Autodesk Inventor part; units mm, degrees
ref_plane "YZ Plane" through (0, 0, 0) normal (1, 0, 0) x (0, 1, 0)
ref_plane "XZ Plane" through (0, 0, 0) normal (0, 1, 0) x (-1, 0, 0)
ref_plane "XY Plane" through (0, 0, 0) normal (0, 0, 1) x (1, 0, 0)
sketch "Sketch1" plane through (0, 0, 0) normal (0, 1, 0) x (-1, 0, 0)
  line L0 (0, 0) -> (-165, 0)
  line L1 (-165, 0) -> (-165, 100)
  line L2 (0, 0) -> (0, 100)
  line L3 (0, 100) -> (-165, 100)
  dimension "d0" = 165
  dimension "d1" = 100
extrude "Extrusion1" add sketch "Sketch1" along normal blind 3
chamfer "Chamfer1" distance 2 angle 45 4 edges at (165, 1.5, 100) (165, 1.5, 0) (0, 1.5, 100) (0, 1.5, 0)
sketch "Sketch2" plane through (0, 0, 0) normal (0, -1, 0) x (1, 0, 0)
  line L0 (163, 100) -> (165, 98)
  line L1 (165, 98) -> (135, 98)
  line L2 (135, 98) -> (135, 74.7)
  line L3 (135, 98) -> (90, 98)
  line L4 (135, 74.7) -> (90, 74.7)
  line L5 (90, 74.7) -> (90, 98)
  line L6 (89, 73.7) -> (136, 73.7)
  line L7 (136, 73.7) -> (136, 99)
  line L8 (136, 99) -> (89, 99)
  line L9 (89, 99) -> (89, 73.7)
  line L10 (165, 98) -> (165, 2)
  line L11 (165, 2) -> (135, 2)
  line L12 (135, 2) -> (135, 25.3)
  line L13 (135, 25.3) -> (90, 25.3)
  line L14 (90, 25.3) -> (90, 2)
  line L15 (90, 2) -> (135, 2)
  line L16 (136, 26.3) -> (136, 1)
  line L17 (136, 1) -> (89, 1)
  line L18 (89, 1) -> (89, 26.3)
  line L19 (89, 26.3) -> (136, 26.3)
  point P0 (0, 0)
  dimension "d7" = 30
  dimension "d8" = 23.3
  dimension "d9" = 45
  dimension "d10" = 1
  dimension "d11" = 23.3
  dimension "d12" = 1
  dimension "d24" = 45
extrude "Extrusion2" add sketch "Sketch2" along normal blind 50 contours L2 L4 L5 L3 | L7 L6 L9 L8 | L15 L14 L13 L12 | L16 L17 L18 L19
sketch "Sketch3" plane through (136, 0, 99) normal (1, 0, 0) x (0, 0, -1)
  line L0 (72.7, 0) -> (72.7, -50)
  line L1 (72.7, -50) -> (72.7, -23)
  line L2 (72.7, -23) -> (98, -23)
  line L3 (98, 0) -> (98, -50)
  line L4 (98, -23) -> (98, -50)
  line L5 (98, -50) -> (72.7, -50)
  line L6 (96, -25) -> (74.7, -25)
  line L7 (74.7, -25) -> (74.7, -48)
  line L8 (74.7, -48) -> (96, -48)
  line L9 (96, -48) -> (96, -25)
  line L10 (25.3, 0) -> (25.3, -50)
  line L11 (0, -50) -> (25.3, -50)
  line L12 (25.3, -50) -> (25.3, -23)
  line L13 (25.3, -23) -> (0, -23)
  line L14 (0, -23) -> (0, -50)
  line L15 (2, -25) -> (23.3, -25)
  line L16 (23.3, -25) -> (23.3, -48)
  line L17 (23.3, -48) -> (2, -48)
  line L18 (2, -48) -> (2, -25)
  point P0 (99, 0)
  dimension "d15" = 27
  dimension "d16" = 2
  dimension "d17" = 2
extrude "Extrusion3" cut sketch "Sketch3" against normal blind 45.5 contours L9 L8 L7 L6 | L15 L16 L17 L18
sketch "Sketch4" plane through (89, 0, 1) normal (-1, 0, 0) x (0, 0, 1)
  circle A0 centre (12.65, -37.966) radius 2.5
  circle A1 centre (85.35, -40.466) radius 2.5
  point P0 (-1, 0)
  dimension "d20" = 5
  dimension "d21" = 5
extrude "Extrusion4" cut sketch "Sketch4" against normal blind 41
sketch "Sketch5" plane through (0, 0, 0) normal (0, -1, 0) x (1, 0, 0)
  line L0 (89, 1) -> (89, 26.3)
  line L1 (89, 73.7) -> (89, 99)
  line L2 (42.1762, 44) -> (98.4238, 44)
  line L3 (70.3, 44) -> (70.3, 56)
  line L4 (70.3, 56) -> (59, 56)
  line L5 (70.3, 56) -> (81.6, 56)
  line L6 (81.6, 56) -> (81.6, 44)
  line L7 (59, 56) -> (59, 44)
  line L8 (59, 50) -> (35, 50)
  line L9 (35, 50) -> (35, 12)
  line L10 (35, 50) -> (35, 88)
  circle A0 centre (35, 12) radius 3.1
  circle A1 centre (35, 88) radius 3.1
  line L11 (89, 73.7) -> (136, 73.7)
  line L12 (89, 73.7) -> (71, 73.7)
  point P0 (0, 0)
  point P1 (65, 50)
  point P2 (71, 50)
  point P3 (53.7, 50)
  dimension "d25" = 12
  dimension "d26" = 11.3
  dimension "d27" = 11.3
  dimension "d28" = 24
  dimension "d29" = 38
  dimension "d30" = 38
  dimension "d31" = 6.2
  dimension "d32" = 6.2
  dimension "d39" = 18
extrude "Extrusion5" cut sketch "Sketch5" against normal blind 45.5
sketch "Sketch6" plane through (0, 3, 0) normal (0, 1, 0) x (1, 0, 0)
  line L0 (59, -44) -> (81.6, -44)
  line L1 (70.3, -44) -> (70.3, -27.55)
  line L2 (70.3, -44) -> (86.75, -44)
  line L3 (86.75, -44) -> (86.75, -56)
  line L4 (86.75, -56) -> (70.3, -56)
  line L5 (70.3, -56) -> (70.3, -27.55)
  point P0 (0, 0)
  point P1 (71, -38.7)
  dimension "d35" = 16.45
  dimension "d36" = 16.45
extrude "Extrusion6" cut sketch "Sketch6" against normal blind 2.1
sketch "Sketch7" plane through (0, 3, 0) normal (0, 1, 0) x (1, 0, 0)
  line L0 (81.6, -44) -> (59, -44)
  line L1 (70.3, -44) -> (54.05, -44)
  line L2 (70.3, -44) -> (86.55, -44)
  line L3 (54.05, -44) -> (54.05, -56)
  line L4 (86.75, -56) -> (81.6, -56)
  line L5 (54.05, -56) -> (86.75, -56)
  line L6 (86.75, -56) -> (86.55, -44)
  point P0 (0, 0)
  dimension "d40" = 16.25
  dimension "d41" = 16.25
extrude "Extrusion7" cut sketch "Sketch7" against normal blind 2
sketch "Sketch8" plane through (0, 0, 0) normal (0, -1, 0) x (1, 0, 0)
  line L0 (0, 2) -> (0, 98)
  line L1 (0, 50) -> (3, 50)
  line L2 (3, 50) -> (3, 60)
  line L3 (2, 100) -> (163, 100)
  line L4 (3, 50) -> (3, 40)
  line L5 (3, 40) -> (8, 40)
  line L6 (8, 40) -> (8, 60)
  line L7 (8, 60) -> (3, 60)
  line L8 (10, 62) -> (10, 38)
  line L9 (10, 38) -> (1, 38)
  line L10 (1, 38) -> (1, 50)
  line L11 (1, 50) -> (1, 62)
  line L12 (1, 62) -> (10, 62)
  point P0 (0, 0)
  dimension "d44" = 3
  dimension "d45" = 10
  dimension "d46" = 10
  dimension "d47" = 5
  dimension "d48" = 2
extrude "Extrusion8" add sketch "Sketch8" along normal blind 10
sketch "Sketch9" plane through (89, 0, 99) normal (0, 0, 1) x (1, 0, 0)
  line L0 (47, 0) -> (0, 0)
  line L1 (23.5, 0) -> (28.5, 0)
  line L2 (23.5, 0) -> (18.5, 0)
  line L3 (18.5, 0) -> (18.5, -10)
  line L4 (18.5, -10) -> (28.5, -10)
  line L5 (28.5, -10) -> (28.5, 0)
  point P0 (-89, 0)
  dimension "d51" = 5
  dimension "d52" = 5
  dimension "d53" = 10
extrude "Extrusion9" add sketch "Sketch9" along normal blind 10
sketch "Sketch10" plane through (107.5, 0, 100) normal (0, 1, 0) x (1, 0, 0)
  line L0 (0, 0) -> (0, -9)
  line L1 (10, 0) -> (10, -9)
  line L2 (0, 0) -> (10, 0)
  line L3 (10, 0) -> (10, -9)
  line L4 (10, -9) -> (0, -9)
  line L5 (0, -9) -> (0, 0)
  line L6 (1.5, -7.5) -> (8.5, -7.5)
  line L7 (8.5, -7.5) -> (8.5, -1.5)
  line L8 (8.5, -1.5) -> (1.5, -1.5)
  line L9 (1.5, -1.5) -> (1.5, -7.5)
  point P0 (-107.5, 100)
  dimension "d56" = 1.5
extrude "Extrusion10" cut sketch "Sketch10" against normal blind 8.5 contours L9 L8 L7 L6
sketch "Sketch11" plane through (136, 0, 1) normal (0, 0, -1) x (-1, 0, 0)
  line L0 (28.5, 0) -> (28.5, -10)
  line L1 (28.5, 0) -> (28.5, -10)
  line L2 (18.5, -10) -> (18.5, 0)
  line L3 (28.5, -10) -> (18.5, -10)
  line L4 (18.5, -10) -> (18.5, 0)
  line L5 (28.5, 0) -> (18.5, 0)
  point P0 (136, 0)
extrude "Extrusion11" add sketch "Sketch11" along normal blind 10
sketch "Sketch12" plane through (107.5, 0, 0) normal (0, 1, 0) x (1, 0, 0)
  line L0 (10, 0) -> (0, 0)
  line L1 (0, 0) -> (0, 9)
  line L2 (0, 0) -> (0, 9)
  line L3 (10, 0) -> (10, 9)
  line L4 (0, 9) -> (10, 9)
  line L5 (10, 9) -> (10, 0)
  line L6 (10, 0) -> (0, 0)
  line L7 (8.5, 7.5) -> (1.5, 7.5)
  line L8 (1.5, 7.5) -> (1.5, 1.5)
  line L9 (1.5, 1.5) -> (8.5, 1.5)
  line L10 (8.5, 1.5) -> (8.5, 7.5)
  point P0 (-107.5, 0)
  dimension "d61" = 1.5
extrude "Extrusion12" cut sketch "Sketch12" against normal blind 8.5 contours L10 L9 L8 L7
sketch "Sketch13" plane through (0, 3, 0) normal (0, 1, 0) x (1, 0, 0)
  circle A0 centre (112.58, -50) radius 2.5
  point P0 (0, 0)
  dimension "d64" = 5
extrude "Extrusion13" cut sketch "Sketch13" against normal blind 8.5
sketch "Sketch14" plane through (0, 0, 0) normal (0, -1, 0) x (1, 0, 0)
  line L0 (165, 98) -> (165, 2)
  line L1 (165, 50) -> (162, 50)
  line L2 (162, 50) -> (162, 40)
  line L3 (162, 50) -> (162, 60)
  line L4 (162, 40) -> (157, 40)
  line L5 (157, 40) -> (157, 60)
  line L6 (157, 60) -> (162, 60)
  line L7 (155, 38) -> (164, 38)
  line L8 (164, 38) -> (164, 50)
  line L9 (164, 50) -> (164, 62)
  line L10 (164, 62) -> (155, 62)
  line L11 (155, 62) -> (155, 38)
  point P0 (0, 0)
  dimension "d67" = 3
  dimension "d68" = 10
  dimension "d69" = 10
  dimension "d70" = 5
  dimension "d71" = 2
extrude "Extrusion14" add sketch "Sketch14" along normal blind 10
properties part number "DesainV1.3"
Input: part model. Units: mm. Frame: model coordinates. A direction names the side the tool comes from. Round coordinates to 2 decimals unless told otherwise and drop trailing zeros. Loops run counter-clockwise (first coordinate to the right, second up) from the corner with the lowest first, then second, coordinate; pieces in that order, holes last. Notation, with made-up numbers: (58.25, -18) - (86.25, -18) arc R24 ccw to (86.25, 18) - close; hole circle Ø3 at (73, 38). An arc over 180 degrees is marked (long way). One line per item, written item: value. Start each with the question number.
(1) Section D-D, the plane x = 67.5. Return loops of the section in (y, z).
(2) Ray query, line 1 (Z direction, x = 132.5, y = -46.5); line 2 (X direction, y = -3, z = 57); line 3 (Z direction, x = 97, y = -20). Return the intervals inside material, ascending. Write a range as [from, to].
(3) Section C-C, the plane x = 130.5. Return loops of the section in (y, z), plus the area to 3 significant figures.
(4) Contact query for flat-ended pins moving along their axis: P1, Ø3, axis at x = 47.5, z = 63, coming from the -Y side; P2, Ø1, axis at x = 137.5, y = -36.5, coming from the +Z side (1 decimal); P3, Ø3, axis at x = 120, y = -17.5, coming from the +Z side; P4, Ø6.5, axis at y = -37.966, z = 13.65, coming from the +X side. Output: stop coordinate, or through.
(5) Draft query along Y for faces 5 (the flat face through (114, -25, 14)), 6 (the flat face through (84, 0.9, 50)), 7 (the flat face through (112, -25, 73.7)). Return one class per face: +Y half, -Y half, draft (parallel to the pull), parting line (faces both ways), or undercut.
(6) Access query for faces 1 (the flat face through (6, -5, 38)), 2 (the flat face through (89, -25, 13)), 3 (the flat face through (112, -10, 104)), 4 (the flat face through (90.5, -36, 16)). Directions: +Z, -Z, +X, -X, +Y, -Y. A direction counts if a zero-diameter tool reaches every point of the face in a straight line with its end or side. Return the directions, or none.
(7) Section B-B, the plane y = -18. Return loops of the section in (x, z), plus the area to 3 significant figures.
(8) Section A-A, the plane z = 50. Count the separate pieces of the cut face and the enclosed holes in it, plus the area to 3 significant figures.
Results below:
1. outline: (0, 0) - (3, 0) - (3, 44) - (0, 44) - close; (0, 56) - (3, 56) - (3, 100) - (0, 100) - close
2. line 1: [1, 3], [24.3, 26.3], [73.7, 75.7], [97, 99]
2. line 2: [1, 3], [8, 10], [155, 157], [162, 164]
2. line 3: [1, 26.3], [73.7, 99]
3. outline: (-50, 1) - (0, 1) - (0, 0) - (3, 0) - (3, 100) - (0, 100) - (0, 99) - (-50, 99) - (-50, 73.7) - (0, 73.7) - (0, 26.3) - (-50, 26.3) - close; hole (-48, 3) - (-25, 3) - (-25, 24.3) - (-48, 24.3) - close; hole (-48, 75.7) - (-25, 75.7) - (-25, 97) - (-48, 97) - close
3. area: 1,850 mm^2
4. P1: y = 0
4. P2: through
4. P3: z = 99
4. P4: x = 90.5
5. face 5: undercut
5. face 6: +Y half
5. face 7: draft
6. face 1: -Z, +X, -X, -Y
6. face 2: +Z, -Z, -X, -Y
6. face 3: +Z, +X, -X, -Y
6. face 4: +X
7. outline: (89, 1) - (136, 1) - (136, 26.3) - (89, 26.3) - close; (89, 73.7) - (136, 73.7) - (136, 99) - (89, 99) - close
7. area: 2,380 mm^2
8. separate pieces: 3
8. enclosed holes: 0
8. area: 471 mm^2
